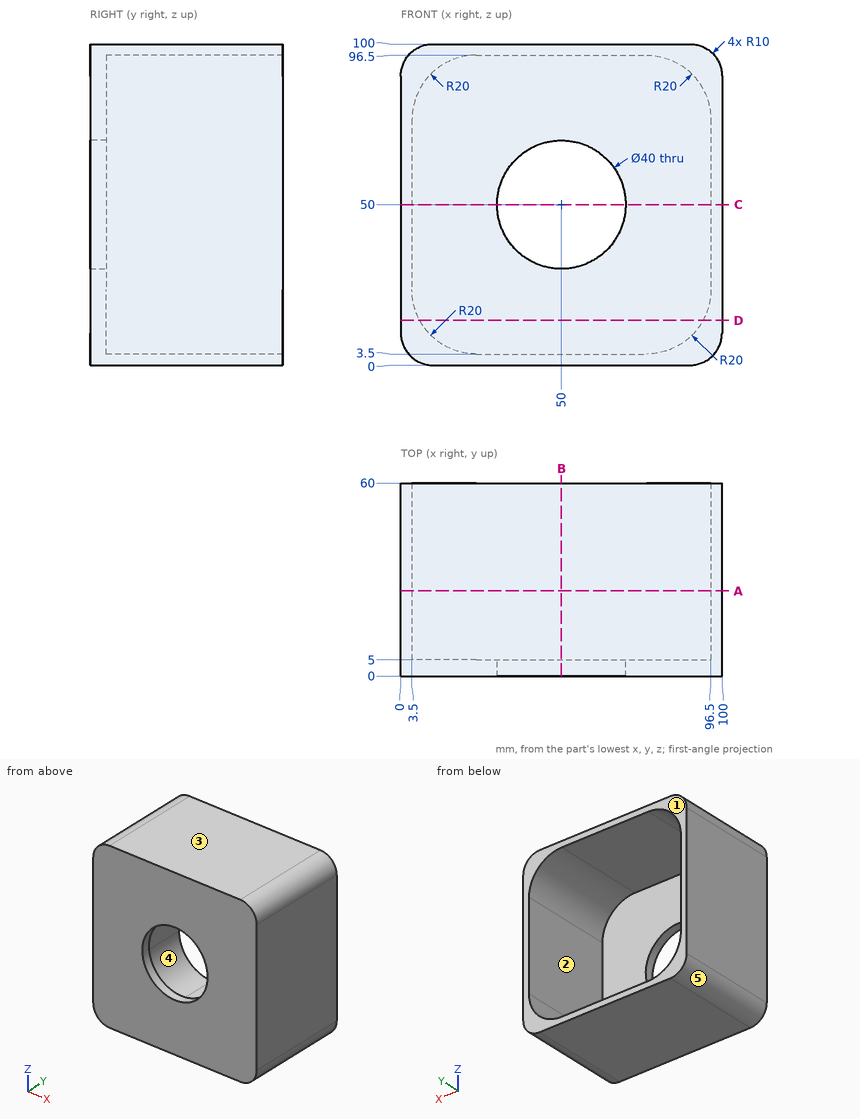
Verification items for this drawing (mm, ordinates from the low corner). A direction names the side the tool comes from. Round coordinates to 2 decimals unless told otherwise and drop trailing zeros. Order: outer loops, then holes, each group sorted by start corner. A loop starts at its lowest first (then second) coordinate and runs counter-clockwise, first axis right, second up. Notation, with made-up numbers: (35.25, 9.25) - (81.25, 9.25) arc R23 cw to (81.25, 28.25) - close; hole circle Ø1 at (10.5, 6.5). An arc over 180 degrees is marked (long way). Use CSV: the item, a comma, the result in double quotes. Start each with the question number.
1) Section check C-C, the plane z = 50. Record the cut outline in (x, y).
2) Go/stop test with a flat-tipped pin: P1, Ø4, axis at x = 43.5, z = 72, coming from the +Y side. Record where the tip stops, or that it passes through.
3) Access from +Z, -Z, +X, -X, +Y, -Y to the whole of each face (thin tool, end or side, straight path). Record for the marked faces 1 and 2.
4) Section check B-B, the plane x = 50. Record the cut outline in (y, z), plus the area to 3 significant figures.
5) Thickness scan on L1, parallel to X at y = 19.5, z = 57; L2, parallel to X at y = 3.7, z = 50. Record the ranges inside material, lowest first.
6) Mould release check, pull along X, two halves, no side actions. Record for the marked faces 3, 4 and 5: +X half, -X half, draft (parallel to the pull), parting line (faces both ways), or undercut.
7) Section check D-D, the plane z = 14. Record the cut outline in (x, y), plus the area to 3 significant figures.
8) Section check A-A, the plane y = 26.5. Record the cut outline in (x, z).
Answers:
1,outline,"(0, 0) - (30, 0) - (30, 5) - (3.5, 5) - (3.5, 60) - (0, 60) - close; (70, 0) - (100, 0) - (100, 60) - (96.5, 60) - (96.5, 5) - (70, 5) - close"
2,P1,"stops at y = 5"
3,face 1,"+Z, -Z, +X, -X, +Y"
3,face 2,"+Y"
4,outline,"(0, 0) - (60, 0) - (60, 3.5) - (5, 3.5) - (5, 30) - (0, 30) - close; (0, 70) - (5, 70) - (5, 96.5) - (60, 96.5) - (60, 100) - (0, 100) - close"
4,area,"685 mm²"
5,L1,"x = 0 to 3.5, 96.5 to 100"
5,L2,"x = 0 to 30, 70 to 100"
6,face 3,"draft"
6,face 4,"undercut"
6,face 5,"-X half"
7,outline,"(0, 0) - (100, 0) - (100, 60) - (94.1, 60) - (94.1, 5) - (5.9, 5) - (5.9, 60) - (0, 60) - close"
7,area,"1,150 mm²"
8,outline,"(0, 10) arc R10 ccw to (10, 0) - (90, 0) arc R10 ccw to (100, 10) - (100, 90) arc R10 ccw to (90, 100) - (10, 100) arc R10 ccw to (0, 90) - close; hole (3.5, 23.5) arc R20 ccw to (23.5, 3.5) - (76.5, 3.5) arc R20 ccw to (96.5, 23.5) - (96.5, 76.5) arc R20 ccw to (76.5, 96.5) - (23.5, 96.5) arc R20 ccw to (3.5, 76.5) - close"
